from build123d import *

# Parameters (mm, degrees)
SKETCH2_W           = 30
SKETCH2_H           = 14
BOSS_EXTRUDE1_DEPTH = 10
SKETCH3_R           = 7
BOSS_EXTRUDE2_DEPTH = 40


with BuildPart() as part:
    # Sketch2 → Boss-Extrude1 (new body)
    with BuildSketch(Plane(origin=(0, 0, 0), x_dir=(1, 0, 0), z_dir=(0, 1, 0))):
        Rectangle(SKETCH2_W, SKETCH2_H)
    extrude(amount=-BOSS_EXTRUDE1_DEPTH)

    # Sketch3 → Boss-Extrude2 (add)
    with BuildSketch(Plane.XZ.offset(10)):
        Circle(SKETCH3_R)
    extrude(amount=BOSS_EXTRUDE2_DEPTH)


solid = part.part
For this review, take the finished solid that the model builds, in its own axes (mm). A direction names the side the tool comes from. Coordinates: 2 decimals unless noted, no trailing zeros. Order: outer loops, then holes, each group sorted by start corner. A loop starts at its lowest first (then second) coordinate and runs counter-clockwise, first axis right, second up. Notation, with made-up numbers: (-27, 56) - (16, 56) arc R23 cw to (16, 85) - close; hole circle Ø11 at (27.25, -7). An arc over 180 degrees is marked (long way). Answer as CSV lines item,"result". Start each with the question number.
1) Add section D-D (x = 11.75). State the section outline as (y, z) points.
2) Add section A-A (z = 0). State the section outline as (x, y) points.
3) Add section B-B (x = 5.75). State the section outline as (y, z) points.
4) To check wall thickness, follow line 1 along Y through (x, z) = (-13, 5.5); line 2 along X through (y, z) = (-48, -3.5); line 3 along Z through (x, y) = (0.75, -44). State the ranges of each line that lie inside material, in increasing order. Write a range as [from, to].
5) Insertion check: P1, Ø3, axis at y = -16, z = -4.5, coming from the +X side; P2, Ø6, axis at x = 8, y = -33, coming from the -Z side; P3, Ø1.5, axis at x = 2.5, y = -27, coming from the -Z side. Each pin has a flat end and moves straight along its axis. Give the tip position at first contact, or say it passes through.
6) Add section C-C (y = -34). State the section outline as (x, z) points.
7) Machinability: for faces 1 (the cylindrical face through (6.466, -29.72, -2.681)), 2 (the flat face through (0, -50, 0)), which of the approach directions +Z, -Z, +X, -X, +Y, -Y give a long, thin tool a straight path to every point of the face, cutting with its end or side? Answer none if there is none.
Result:
1,outline,"(-10, -7) - (0, -7) - (0, 7) - (-10, 7) - close"
2,outline,"(-15, -10) - (-7, -10) - (-7, -50) - (7, -50) - (7, -10) - (15, -10) - (15, 0) - (-15, 0) - close"
3,outline,"(-50, -3.99) - (-10, -3.99) - (-10, -7) - (0, -7) - (0, 7) - (-10, 7) - (-10, 3.99) - (-50, 3.99) - close"
4,line 1,"[-10, 0]"
4,line 2,"[-6.06, 6.06]"
4,line 3,"[-6.96, 6.96]"
5,P1,"x = 6.32"
5,P2,"z = -4.9"
5,P3,"z = -6.78"
6,outline,"circle Ø14 at (0, 0)"
7,face 1,"-Y"
7,face 2,"+Z, -Z, +X, -X, -Y"
